Geometry: final body of the model. Coordinates: model frame, mm. Round coordinates to 2 decimals unless told otherwise and drop trailing zeros. Order: outer loops, then holes, each group sorted by start corner. A loop starts at its lowest first (then second) coordinate and runs counter-clockwise, first axis right, second up. Notation, with made-up numbers: M 32.5,35 L 64.5,35 A19 ccw 64.5,53 Z; hole C 64,61.5 d1. An arc over 180 degrees is marked long. Put each result on its own line as item: value. Start each with the question number.
1) Draft query along Y for faces 1 (the cylindrical face through (-61.69, -23.49, 0.01)), 2 (the flat face through (-1, 0, -2.277)), 3 (the cylindrical face through (46.44, 0.19, -0.03)). Return one class per face: pulls with the +Y half, pulls with the -Y half, needs draft (parallel to the pull), parting line crosses it, or undercut.
2) Section A-A, the plane y = 0. Return loops of the section in (x, z) (1 decimal).
3) Section C-C, the plane z = 1.4. Return loops of the section in (x, y), then the cut area to 3 significant figures.
4) Material intervals for probe 1 along X at (y, z) = (-4, 0.45); probe 2 along X at (y, z) = (-3, 1.1); probe 3 along Y at (x, z) = (31.75, 0.75), sorted ascending. Write a range as [from, to].
5) Section D-D, the plane x = 50.8. Return loops of the section in (y, z) (1 decimal), then the cut area to 3 significant figures.
from build123d import *

# Parameters (mm, degrees)
F0_R     = 4.365625
F0_R_2   = 6.35
F1_DEPTH = 2.27711
F2_R     = 1.5875


with BuildPart() as f1:
    # F0 (on Top) → F1 (new body, symmetric)
    with BuildSketch(Plane.XY):
        with BuildLine():
            Line((57.15, 25.4), (-57.15, 25.4))
            ThreePointArc((-57.15, 25.4), (-61.640128, 23.540128), (-63.5, 19.05))
            Line((-63.5, 19.05), (-63.5, -19.05))
            ThreePointArc((-63.5, -19.05), (-61.640128, -23.540128), (-57.15, -25.4))
            Line((-57.15, -25.4), (57.15, -25.4))
            ThreePointArc((57.15, -25.4), (61.640128, -23.540128), (63.5, -19.05))
            Line((63.5, -19.05), (63.5, 19.05))
            ThreePointArc((63.5, 19.05), (61.640128, 23.540128), (57.15, 25.4))
        make_face()
        with Locations((-50.8, 0)):
            Circle(F0_R, mode=Mode.SUBTRACT)
        with Locations((-31.75, 0)):
            Circle(F0_R_2, mode=Mode.SUBTRACT)
        with Locations((31.75, 0)):
            Circle(F0_R_2, mode=Mode.SUBTRACT)
        with Locations((50.8, 0)):
            Circle(F0_R, mode=Mode.SUBTRACT)
    extrude(amount=F1_DEPTH, both=True)

    # F2
    f2_edges = [f1.edges().sort_by_distance(p)[0] for p in [
        (0, -25.4, 2.27711),
        (0, -25.4, -2.27711),
    ]]
    fillet(f2_edges, radius=F2_R)


solid = f1.part
Result sheet:
1. face 1: pulls with the -Y half
1. face 2: needs draft
1. face 3: undercut
2. outline: M -63.5,-0.7 A1.6 ccw -61.9,-2.3 L -55.2,-2.3 L -55.2,2.3 L -61.9,2.3 A1.6 ccw -63.5,0.7 Z; M -46.4,-2.3 L -38.1,-2.3 L -38.1,2.3 L -46.4,2.3 Z; M -25.4,-2.3 L 25.4,-2.3 L 25.4,2.3 L -25.4,2.3 Z; M 38.1,-2.3 L 46.4,-2.3 L 46.4,2.3 L 38.1,2.3 Z; M 55.2,-2.3 L 61.9,-2.3 A1.6 ccw 63.5,-0.7 L 63.5,0.7 A1.6 ccw 61.9,2.3 L 55.2,2.3 Z
3. outline: M -63.33,-19.05 A6.18 ccw -57.15,-25.23 L 57.15,-25.23 A6.18 ccw 63.33,-19.05 L 63.33,19.05 A6.18 ccw 57.15,25.23 L -57.15,25.23 A6.18 ccw -63.33,19.05 Z; hole C -50.8,0 d8.73; hole C -31.75,0 d12.7; hole C 31.75,0 d12.7; hole C 50.8,0 d8.73
3. area: 5,990 mm2
4. probe 1: x = [-63.5, -52.55], [-49.05, -36.68], [-26.82, 26.82], [36.68, 49.05], [52.55, 63.5]
4. probe 2: x = [-63.45, -53.97], [-47.63, -37.35], [-26.15, 26.15], [37.35, 47.63], [53.97, 63.45]
4. probe 3: y = [-25.4, -6.35], [6.35, 25.4]
5. outline: M -25.4,-0.7 A1.6 ccw -23.8,-2.3 L -4.4,-2.3 L -4.4,2.3 L -23.8,2.3 A1.6 ccw -25.4,0.7 Z; M 4.4,-2.3 L 23.8,-2.3 A1.6 ccw 25.4,-0.7 L 25.4,0.7 A1.6 ccw 23.8,2.3 L 4.4,2.3 Z
5. area: 189 mm2
